from build123d import *

# Parameters (mm, degrees)
SKETCH1_W           = 4
SKETCH1_H           = 3.5
SKETCH2_R           = 2
BOSS_EXTRUDE1_DEPTH = 45
CUT_EXTRUDE1_DEPTH  = 2
CHAMFER1_SIZE       = 0.4295


with BuildPart() as part:
    # Sketch1 → Revolve1 (revolve)
    with BuildSketch(Plane.XY, mode=Mode.PRIVATE) as revolve1_sk:
        with Locations((-2, 1.75)):
            Rectangle(SKETCH1_W, SKETCH1_H)
    revolve(revolve1_sk.sketch.rotate(Axis((-4, 0, 0), (1, 0, 0)), 270), axis=Axis((-4, 0, 0), (1, 0, 0)))

    # Sketch2 → Boss-Extrude1 (add)
    with BuildSketch(Plane(origin=(0, 0, 0), x_dir=(0, 0, -1), z_dir=(1, 0, 0))):
        with Locations(Location((0, 0, 0), (0, 0, 180))):
            Circle(SKETCH2_R)
    extrude(amount=BOSS_EXTRUDE1_DEPTH)

    # Sketch3 → Cut-Extrude1 (cut)
    with BuildSketch(Plane.ZY.offset(4)):
        Polygon((1.5, -0.866025404), (1.5, 0.866025404), (0, 1.732050808), (-1.5, 0.866025404), (-1.5, -0.866025404), (0, -1.732050808), align=None)
    extrude(amount=-CUT_EXTRUDE1_DEPTH, mode=Mode.SUBTRACT)

    # Sketch4 → Cut-Revolve1 (revolve, cut)
    with BuildSketch(Plane.XY, mode=Mode.PRIVATE) as cut_revolve1_sk:
        Polygon((-2, 1.5), (-2, 0), (-1.598076211, 0), align=None)
    revolve(cut_revolve1_sk.sketch.rotate(Axis((-2.000025, 0, 0), (1, 0, 0)), 90), axis=Axis((-2.000025, 0, 0), (1, 0, 0)), mode=Mode.SUBTRACT)

    # Chamfer1
    chamfer1_edges = [part.edges().sort_by_distance(p)[0] for p in [
        (45, 0, -2),
    ]]
    chamfer(chamfer1_edges, length=CHAMFER1_SIZE)


solid = part.part
Check sheet for the modelled part. Datum: model origin and axes. Units: mm. A direction names the side the tool comes from. Round coordinates to 2 decimals unless told otherwise and drop trailing zeros. Order: outer loops, then holes, each group sorted by start corner. A loop starts at its lowest first (then second) coordinate and runs counter-clockwise, first axis right, second up.
(1) Cross-section at B-B, the plane y = -2.75. Enter the section's corners in (x, z), and give its area (3 significant figures).
(2) Scan lines: probe 1 along Y at (x, z) = (30.5, -1.25); probe 2 along Y at (x, z) = (-1.5, 0.25); probe 3 along X at (y, z) = (-1.25, -1.75). Record each from-to range of solid material in increasing order.
(3) Access from +Z, -Z, +X, -X, +Y, -Y to the whole of each face (thin tool, end or side, straight path). Record for faces 4 (the flat face through (-3.014, -1.305, 0.74)), 5 (the flat face through (-4, 0, 2)), 6 (the flat face through (0, -2, 2)).
(4) Cross-section at C-C, the plane z = -3. Enter the section's corners in (x, y).
(5) Cross-section at A-A, the plane x = 22. Enter the section's corners in (y, z).
(6) Draft check along Z on faces 1 (the cylindrical face through (-1.972, -3.417, 0.759)), 2 (the flat face through (-3, 0, -1.5)), 3 (the flat face through (45, 0, 0)). Enter one of: pulls with the +Z half, pulls with the -Z half, needs draft (parallel to the pull), parting line crosses it, or undercut.
(7) Go/stop test with flat-tipped pins: P1, Ø4, axis at x = 18.5, z = -1.5, coming from the +Y side; P2, Ø0.6, axis at y = -0.5, z = -1, coming from the -X side; P3, Ø0.8, axis at y = -1, z = 1, coming from the -X side; P4, Ø1.5, axis at y = -1, z = 2.5, coming from the +X side. Record where each tip stops, or that it passes through.
Check sheet entries:
1. outline: (-4, -2.17) - (0, -2.17) - (0, 2.17) - (-4, 2.17) - close
1. area: 17.3 mm2
2. probe 1: y = -1.56 to 1.56
2. probe 2: y = -3.49 to 3.49
2. probe 3: x = -4 to 0
3. face 4: -X
3. face 5: +Z, -Z, -X, +Y, -Y
3. face 6: +X
4. outline: (-4, -1.8) - (0, -1.8) - (0, 1.8) - (-4, 1.8) - close
5. outline: circle Ø4 at (0, 0)
6. face 1: parting line crosses it
6. face 2: undercut
6. face 3: needs draft
7. P1: stops at y = 2
7. P2: stops at x = -1.98
7. P3: stops at x = -4
7. P4: stops at x = 44.63
